from build123d import *

# Parameters (mm, degrees)
F2_DEPTH = 2
F3_D     = 2
F4_D     = 2
F5_D     = 2
F6_D     = 2
F1_W     = 48.5
F1_H     = 2
F7_DEPTH = 12
F8_SIZE  = 10
F9_SIZE  = 10
F12_D    = 3.25


with BuildPart() as f2:
    # F0 (on Front) → F2 (new body)
    with BuildSketch(Plane.XZ):
        Polygon((-24.25, 11.75), (-24.25, -13.75), (24.25, -13.75), (24.25, 11.75), (5.5228731483, 11.75), (5.5228731483, 5.75), (-6.4771268517, 5.75), (-6.4771268517, 11.75), align=None)
    extrude(amount=F2_DEPTH)

    # F3 (through all)
    with Locations(Plane(origin=(0, 0, 0), x_dir=(1, 0, 0), z_dir=(0, 1, 0))):
        with Locations((-21.25, -8.75)):
            Hole(F3_D / 2)

    # F4 (through all)
    with Locations(Plane(origin=(0, 0, 0), x_dir=(1, 0, 0), z_dir=(0, 1, 0))):
        with Locations((-21.25, 8.75)):
            Hole(F4_D / 2)

    # F5 (through all)
    with Locations(Plane(origin=(0, 0, 0), x_dir=(1, 0, 0), z_dir=(0, 1, 0))):
        with Locations((21.25, -8.75)):
            Hole(F5_D / 2)

    # F6 (through all)
    with Locations(Plane(origin=(0, 0, 0), x_dir=(1, 0, 0), z_dir=(0, 1, 0))):
        with Locations((21.25, 8.75)):
            Hole(F6_D / 2)

    # F1 (on Front) → F7 (join)
    with BuildSketch(Plane.XZ):
        with Locations((0, -14.75)):
            Rectangle(F1_W, F1_H)
    extrude(amount=F7_DEPTH)

    # F8
    f8_edges = [f2.edges().sort_by_distance(p)[0] for p in [
        (24.25, -12, -14.75),
    ]]
    chamfer(f8_edges, length=F8_SIZE)

    # F9
    f9_edges = [f2.edges().sort_by_distance(p)[0] for p in [
        (-24.25, -12, -14.75),
    ]]
    chamfer(f9_edges, length=F9_SIZE)

    # F12 (through all)
    with Locations(Plane(origin=(0, 0, -15.75), x_dir=(1, 0, 0), z_dir=(0, 0, -1))):
        with Locations((0, 7)):
            Hole(F12_D / 2)


solid = f2.part
Can you work these out from the model? Positions are in its coordinate system, mm. A direction names the side the tool comes from. Coordinates: 2 decimals unless noted, no trailing zeros. Order: outer loops, then holes, each group sorted by start corner. A loop starts at its lowest first (then second) coordinate and runs counter-clockwise, first axis right, second up. Notation, with made-up numbers: (2, -1) - (32, -1) arc R20 ccw to (32, 25) - close; hole circle Ø2 at (8, -33.75). An arc over 180 degrees is marked (long way). Answer as a JSON object with one key per item and string values. Group by question number.
Q1. Imagine slicing it at A-A (z = -8.75). Please give me the cut outline in (x, y), and give its area (3 significant figures).
Q2. Imagine slicing it at C-C (y = -7). Please give me the cut outline in (x, z) (3 decimals), and give its area (3 significant figures).
Q3. On a 3-axis mill with a long thin cutter (end or side, diameter ignored), from which of +Z, -Z, +X, -X, +Y, -Y can I reach the whole of each face in a straight line? I mean faces 5 (the face through (5.523, -1, 9)), 6 (the face through (0, -2, -1)), 7 (the face through (21.38, -1.01, -9.74)). Say none if no direction works.
Q4. We'd pull the mould along X, two halves only. Please class faces 1 (the face through (-6.477, -1, 9)), 2 (the face through (24.25, -1, -2)), 3 (the face through (0, -5, -15.75)), 4 (the face through (0.21, -8.61, -14.74)): +X half, -X half, draft (parallel to the pull), parting line (faces both ways), or undercut.
Q5. Will these pins go through, and if not, where does the flat tip stop? P1, Ø1.9, axis at x = 0, y = -7, coming from the +Z side; P2, Ø4, axis at x = -1, y = -8, coming from the +Z side; P3, Ø7.5, axis at x = -2.5, z = -7, coming from the -Y side; P4, Ø1, axis at x = -1, y = -1.5, coming from the +Z side.
Q6. Imagine slicing it at D-D (x = 0). Please give me the cut outline in (y, z) (3 decimals), and give its area (3 significant figures).
Q7. Imagine slicing it at B-B (x = 21.25). Please give me the cut outline in (y, z).
Q8. I need wall thicknesses on line 1 (Z direction, x = 21.25, y = -1.4); line 2 (X direction, y = -0.85, z = 8.75); line 3 (X direction, y = -0.9, z = -8.75). Which ranges of each line are inside material? Lowest first, please. Write a range as from..to.
Determined:
{
 "1": {"outline": "(-24.25, -2) - (-22.25, -2) - (-22.25, 0) - (-24.25, 0) - close; (-20.25, -2) - (20.25, -2) - (20.25, 0) - (-20.25, 0) - close; (22.25, -2) - (24.25, -2) - (24.25, 0) - (22.25, 0) - close", "area": "89.0 mm2"},
 "2": {"outline": "(-19.25, -15.75) - (-1.625, -15.75) - (-1.625, -13.75) - (-19.25, -13.75) - close; (1.625, -15.75) - (19.25, -15.75) - (19.25, -13.75) - (1.625, -13.75) - close", "area": "70.5 mm2"},
 "3": {"face 5": "+Z, +Y, -Y", "face 6": "+Z, +X, -X, -Y", "face 7": "+Y, -Y"},
 "4": {"face 1": "undercut", "face 2": "+X half", "face 3": "draft", "face 4": "undercut"},
 "5": {"P1": "passes through", "P2": "stops at z = -13.75", "P3": "stops at y = -2", "P4": "stops at z = 5.75"},
 "6": {"outline": "(-12, -15.75) - (-8.625, -15.75) - (-8.625, -13.75) - (-12, -13.75) - close; (-5.375, -15.75) - (0, -15.75) - (0, 5.75) - (-2, 5.75) - (-2, -13.75) - (-5.375, -13.75) - close", "area": "56.5 mm2"},
 "7": {"outline": "(-5, -15.75) - (0, -15.75) - (0, -9.75) - (-2, -9.75) - (-2, -13.75) - (-5, -13.75) - close; (-2, -7.75) - (0, -7.75) - (0, 7.75) - (-2, 7.75) - close; (-2, 9.75) - (0, 9.75) - (0, 11.75) - (-2, 11.75) - close"},
 "8": {"line 1": "z = -15.75..-9.75, -7.75..7.75, 9.75..11.75", "line 2": "x = -24.25..-22.25, -20.25..-6.48, 5.52..20.25, 22.25..24.25", "line 3": "x = -24.25..-22.25, -20.25..20.25, 22.25..24.25"}
}
